Autodesk Inventor part; units mm, degrees
ref_plane "Work Plane1" through (8, 0, 0) normal (0, 0, -1) x (1, 0, 0)
ref_plane "YZ Plane" through (0, 0, 0) normal (1, 0, 0) x (0, 1, 0)
ref_plane "XZ Plane" through (0, 0, 0) normal (0, 1, 0) x (-1, 0, 0)
sketch "Skizze1" plane through (0, 0, 0) normal (0, 0, 1) x (1, 0, 0)
  line L0 (0, 0) -> (11, 0)
  line L1 (11, 0) -> (11, 2)
  line L2 (11, 2) -> (5, 2)
  line L3 (5, 2) -> (5, 2.75)
  line L4 (5, 2.75) -> (0, 2.75)
  line L5 (0, 2.75) -> (0, 0)
  line L6 (-2.2, 0) -> (13.2, 0)
  line L7 (0, -0.55) -> (0, 3.3)
  arc A0 (5, 2) -> (5.6, 2) centre (5.3, 2.5196) ccw
  dimension "d0" = 5
  dimension "d1" = 6
  dimension "d2" = 4
  dimension "d3" = 5.5
  dimension "d14" = 0.6
  dimension "d15" = 0.6
revolve "Körper" add sketch "Skizze1" angle 360 about axis through (0, 0, 0) along (1, 0, 0)
sketch "Skizze2" plane through (0, 0, 0) normal (-1, 0, 0) x (0, 0, 1)
  circle A0 centre (0, 0) radius 2.75
  line L0 (0, -3.85) -> (0, 3.85)
  line L1 (-3.85, 0) -> (3.85, 0)
  line L2 (-2.75, 0.3) -> (2.75, 0.3)
  line L3 (2.75, 0.3) -> (2.75, -0.3)
  line L4 (2.75, -0.3) -> (-2.75, -0.3)
  line L5 (-2.75, -0.3) -> (-2.75, 0.3)
  line L6 (-2.75, 0) -> (2.75, 0) construction
  line L7 (0, 0.3) -> (0, -0.3) construction
  dimension "d5" = 0.6
extrude "Loch" cut sketch "Skizze2" against normal blind 1.42 contours L1 L0 L2 A0 | L3 L4 A0 | A0 L4 L0 L1 | A0 L2 L3 | L1 A0 L2 L0 | L0 L4 A0 L1 | L5 L2 A0 | A0 L4 L5
chamfer "Fase1" distance 0.8 angle 45 3 edges at (0, 2.0479, -1.8354) (0, 2.0479, 1.8354) (0, -2.75, 0) measured on face at (2.14, 0.7465, 2.6467)
thread "Gewinde"
chamfer "Fase2" distance 0.4294 distance2 0.4294 1 edges at (11, -2, 0) measured on face at (11, 0.6473, 0.1595)
revolve "Nut1" cut sketch "Skizze1" angle 360 about axis through (0, 0, 0) along (1, 0, 0) contours A0 L2
ref_plane "Work Plane1" through (8, 0, 0) normal (0, 0, -1) x (1, 0, 0)
equation "\"d0\" = KOH"
equation "\"d1\" = GEL"
equation "\"d2\" = NND"
equation "\"d3\" = KOD"
equation "\"d14\" = SBR"
equation "\"d15\" = SBR"
equation "\"d5\" = SBR"
equation "\"d6\" = STI"
equation "\"d8\" = PHH"
equation "\"d19\" = PHH"
equation "\"d10\" = GEL"
equation "\"d12\" = -0.5 * GD1 + 0.5 * NND"
equation "\"d13\" = GUL"
equation "\"NND\" = 4"
equation "\"GEL\" = 6"
equation "\"KOD\" = 5.5"
equation "\"KOH\" = 5"
equation "\"SBR\" = 0.6"
equation "\"GUL\" = 0.61345 * PTC"
equation "\"PHH\" = 0.8"
equation "\"GD1\" = THREADDIA - 1.2269 * PTC"
equation "\"STI\" = 1.42"
equation "\"THREADDIA\" = 4"
equation "\"TOA\" = 30deg"
equation "\"NLG\" = GEL"
equation "\"PTC\" = 0.7"
equation "\"GAL\" = 0.61345 * PTC"
properties part number "DIN 927 - M4 x 5-14H" material "Stahl, weich"
CAD build for the part. Positions are in the model's coordinates, mm. A direction names the side the tool comes from. Round coordinates to 2 decimals unless told otherwise and drop trailing zeros. Loops run counter-clockwise (first coordinate to the right, second up) from the corner with the lowest first, then second, coordinate; pieces in that order, holes last. Notation, with made-up numbers: M -4,42 L 21,42 A33 ccw 21,78 Z; hole C 43.25,23 d4. An arc over 180 degrees is marked long. Return JSON: item names as keys, results as strings. Group by question number.
(1) Drop flat-ended pins along their axis: P1, Ø1.1, axis at x = 0.5, z = -0.5, coming from the +Y side; P2, Ø1.5, axis at x = 8.5, z = 1, coming from the -Y side. Give the stop position or say it passes through.
(2) Saw through at A-A, the plane y = 0. List the corners of the cut face in (x, z).
(3) Mould opens along Y. For faces 3 (the conical face through (0.14, -2.09, 0.04)), 4 (the flat face through (1, -0.3, 0)), 5 (the flat face through (1, 0.3, 0)), 6 (the cylindrical face through (2.871, -0.358, -2.727)) say: +Y half, -Y half, draft (parallel to the pull), parting line (faces both ways), or undercut.
(4) Saw through at B-B, the plane z = 0. List the corners of the cut face in (x, y), and give its area (3 significant figures).
(5) Tool access for faces 1 (the flat face through (5, 1, -2)), 2 (the flat face through (0, 1, 0)): list every direction of +Z, -Z, +X, -X, +Y, -Y with a clear straight run to the whole face (end or side of a thin tool).
(6) Saw through at C-C, the plane x = 9. List the corners of the cut face in (y, z).
(7) Wall check: probe 1 along Y at (x, z) = (1, 2.3); probe 2 along X at (y, z) = (-1.6, -1.15); probe 3 along X at (y, z) = (-0.1, -2.2). Give the ranges that are in metal, low to high. Write a range as [from, to].
Answer list:
{
 "1": {"P1": "y = 2.75", "P2": "y = -1.98"},
 "2": {"outline": "M 1.42,-2.75 L 5,-2.75 L 5,-2 A0.6 cw 5.6,-2 L 10.57,-2 L 11,-1.57 L 11,1.57 L 10.57,2 L 5.6,2 A0.6 cw 5,2 L 5,2.75 L 1.42,2.75 Z"},
 "3": {"face 3": "-Y half", "face 4": "undercut", "face 5": "undercut", "face 6": "parting line"},
 "4": {"outline": "M 0,-1.95 L 0.8,-2.75 L 5,-2.75 L 5,-2 A0.6 cw 5.6,-2 L 10.57,-2 L 11,-1.57 L 11,1.57 L 10.57,2 L 5.6,2 A0.6 cw 5,2 L 5,2.75 L 0.8,2.75 L 0,1.95 L 0,0.3 L 1.42,0.3 L 1.42,-0.3 L 0,-0.3 Z", "area": "49.8 mm2"},
 "5": {"face 1": "+X", "face 2": "+Z, -Z, -X, +Y, -Y"},
 "6": {"outline": "C 0,0 d4"},
 "7": {"probe 1": "[-1.51, -0.3], [0.3, 1.51]", "probe 2": "[0.02, 5.06], [5.54, 10.6]", "probe 3": "[1.42, 5]"}
}
